For this review, take the finished solid that the model builds, in its own axes (mm). Round coordinates to 2 decimals unless told otherwise and drop trailing zeros. Order: outer loops, then holes, each group sorted by start corner. A loop starts at its lowest first (then second) coordinate and runs counter-clockwise, first axis right, second up. Notation, with made-up numbers: M 19,-37 L 47,-37 A12 ccw 47,-33 Z; hole C 3,46 d7. An arc over 180 degrees is marked long. Answer as a JSON object with one key per item and string values.
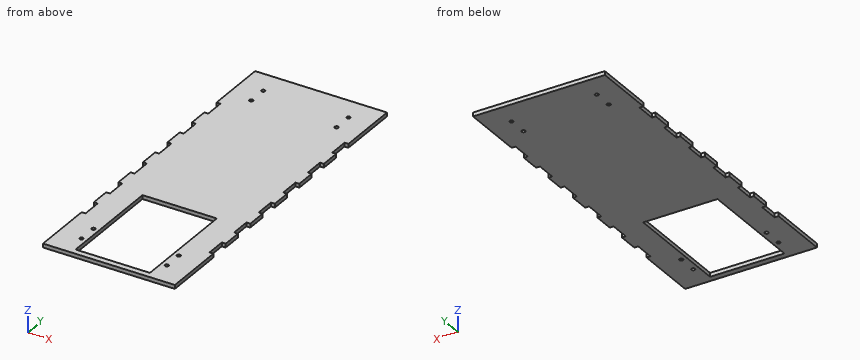
from build123d import *

# Parameters (mm, degrees)
BOSS_EXTRUDE1_DEPTH = 3.175
SKETCH2_R           = 1.5
CUT_EXTRUDE1_DEPTH  = 3.175
SKETCH3_W           = 60.85
SKETCH3_H           = 88.133333333
CUT_EXTRUDE2_DEPTH  = 3.175


with BuildPart() as part:
    # Sketch1 → Boss-Extrude1 (new body)
    with BuildSketch(Plane.XY):
        Polygon((-3.175, 279.4), (-3.175, 228.6), (0, 228.6), (0, 212.436363636), (-3.175, 212.436363636), (-3.175, 196.272727273), (0, 196.272727273), (0, 180.109090909), (-3.175, 180.109090909), (-3.175, 163.945454545), (0, 163.945454545), (0, 147.781818182), (-3.175, 147.781818182), (-3.175, 131.618181818), (0, 131.618181818), (0, 115.454545455), (-3.175, 115.454545455), (-3.175, 99.290909091), (0, 99.290909091), (0, 83.127272727), (-3.175, 83.127272727), (-3.175, 66.963636364), (0, 66.963636364), (0, 50.8), (-3.175, 50.8), (-3.175, 0), (104.775, 0), (104.775, 50.8), (101.6, 50.8), (101.6, 66.963636364), (104.775, 66.963636364), (104.775, 83.127272727), (101.6, 83.127272727), (101.6, 99.290909091), (104.775, 99.290909091), (104.775, 115.454545455), (101.6, 115.454545455), (101.6, 131.618181818), (104.775, 131.618181818), (104.775, 147.781818182), (101.6, 147.781818182), (101.6, 163.945454545), (104.775, 163.945454545), (104.775, 180.109090909), (101.6, 180.109090909), (101.6, 196.272727273), (104.775, 196.272727273), (104.775, 212.436363636), (101.6, 212.436363636), (101.6, 228.6), (104.775, 228.6), (104.775, 279.4), align=None)
    extrude(amount=BOSS_EXTRUDE1_DEPTH)

    # Sketch2 → Cut-Extrude1 (cut)
    with BuildSketch(Plane.XY.offset(3.175)):
        with Locations((15.875, 20)):
            Circle(SKETCH2_R)
        with Locations((15.875, 35.75)):
            Circle(SKETCH2_R)
        with Locations((15.875, 243.65)):
            Circle(SKETCH2_R)
        with Locations((15.875, 259.4)):
            Circle(SKETCH2_R)
        with Locations((85.725, 259.4)):
            Circle(SKETCH2_R)
        with Locations((85.725, 243.65)):
            Circle(SKETCH2_R)
        with Locations((85.725, 35.75)):
            Circle(SKETCH2_R)
        with Locations((85.725, 20)):
            Circle(SKETCH2_R)
    extrude(amount=-CUT_EXTRUDE1_DEPTH, mode=Mode.SUBTRACT)

    # Sketch3 → Cut-Extrude2 (cut)
    with BuildSketch(Plane.XY.offset(3.175)):
        with Locations((50.8, 49.066666667)):
            Rectangle(SKETCH3_W, SKETCH3_H)
    extrude(amount=-CUT_EXTRUDE2_DEPTH, mode=Mode.SUBTRACT)


solid = part.part
1) Add section B-B on y = 24.5. State the section outline as (x, z) points (3 decimals).
Geometry check:
{"outline": "M -3.175,0 L 20.375,0 L 20.375,3.175 L -3.175,3.175 Z; M 81.225,0 L 104.775,0 L 104.775,3.175 L 81.225,3.175 Z"}
2) Add section D-D on y = 224. State the section outline as (x, z) points (3 decimals).
Geometry check:
{"outline": "M 0,0 L 101.6,0 L 101.6,3.175 L 0,3.175 Z"}
3) Add section C-C on z = 2. State how many separate pieces and enclosed holes the cut face has, and give its area (3 significant figures).
Geometry check:
{"separate pieces": "1", "enclosed holes": "9", "area": "24,100 mm²"}
4) Insertion check: P1, Ø2.5, axis at x = 15.875, y = 35.75, coming from the -Z side; P2, Ø1, axis at y = 94, z = 1, coming from the +X side; P3, Ø1, axis at y = 120, z = 2, coming from the -X side. Each pin has a flat end and moves straight along its axis. Give the tip position at first contact, or say it passes through.
Geometry check:
{"P1": "passes through", "P2": "stops at x = 101.6", "P3": "stops at x = 0"}
5) For L1, parallel to X at y = 259.4, z = 0.8 (3 decimals); L2, parallel to Y at x = 65, z = 0.25; L3, parallel to X at y = 56, z = 2.1 (3 decimals), list the stretches that pass through material, from the lowest coordinate up.
Geometry check:
{"L1": "x = -3.175 to 14.375, 17.375 to 84.225, 87.225 to 104.775", "L2": "y = 0 to 5, 93.13 to 279.4", "L3": "x = 0 to 20.375, 81.225 to 101.6"}
6) Add section A-A on x = 29. State the section outline as (y, z) points (3 decimals).
Geometry check:
{"outline": "M 0,0 L 5,0 L 5,3.175 L 0,3.175 Z; M 93.133,0 L 279.4,0 L 279.4,3.175 L 93.133,3.175 Z"}
